```python
from build123d import *

# Parameters (mm, degrees)
F0_R        = 11.05
F1_DEPTH    = 6.5
F2_SIZE     = 2
F3_T1_DEPTH = 28.2168298797


# Not quite as in the source:
# - a fillet or chamfer that OpenCascade refuses, or shapes differently, is made with other operations: its cross-section is extruded or revolved along the edge and cut away or added


with BuildPart() as f1:
    # F0 (on Top) → F1 (new body)
    with BuildSketch(Plane.XY):
        Polygon((30, 0), (30, 15), (-30, 15), (-30, 0), (-30, -15), (30, -15), align=None)
        with BuildLine():
            ThreePointArc((-3.95, 0), (-15, -11.05), (-26.05, 0))
            ThreePointArc((-26.05, 0), (-15, 11.05), (-3.95, 0))
        make_face(mode=Mode.SUBTRACT)
        with Locations((15, 0)):
            Circle(F0_R, mode=Mode.SUBTRACT)
    extrude(amount=F1_DEPTH)

    # F2
    f2_edges = [f1.edges().sort_by_distance(p)[0] for p in [
        (-30, 0, 6.5),
        (-30, 0, 0),
        (0, -15, 0),
        (0, -15, 6.5),
        (0, 15, 0),
        (0, 15, 6.5),
        (30, 0, 0),
        (30, 0, 6.5),
    ]]
    chamfer(f2_edges, length=F2_SIZE)

    # F3: chamfer of 5 on 4 edges, made by hand

    # F3_s2 → F3_t1 (cut)
    with BuildSketch(Plane.XY.offset(-10.8584149398)):
        Polygon((30, 10), (25, 15), (30, 15), align=None)
        Polygon((30, -10), (25, -15), (30, -15), align=None)
        Polygon((-25, 15), (-30, 10), (-30, 15), align=None)
        Polygon((-25, -15), (-30, -10), (-30, -15), align=None)
    extrude(amount=F3_T1_DEPTH, mode=Mode.SUBTRACT)


solid = f1.part
```
For this review, take the finished solid that the model builds, in its own axes (mm). Give positions to 0.01 mm unless a question says otherwise; leave off trailing zeros. Write each loop counter-clockwise with the first axis right and the second up, starting at its lowest first coordinate (ties: lowest second). Pieces come first, ordered by that corner, then holes.
Item 1: Take a section at C-C (z = 5.75). Give the boundary of the cut face in (x, y).
Item 2: Take a section at D-D (y = -5). Give the boundary of the cut face in (x, z).
Item 3: Wall thickness on probe 1 along Y at (x, z) = (-15, 3); probe 2 along X at (y, z) = (-9.5, 5.5); probe 3 along X at (y, z) = (-8, 4.75): over which ranges is each line inside the solid? List them lowest first.
Item 4: Take a section at A-A (y = 0). Give the boundary of the cut face in (x, z), and give its area (3 significant figures).
Item 5: Take a section at B-B (x = -15). Give the boundary of the cut face in (y, z).
Item 6: Insertion check: P1, Ø1.5, axis at x = -5.5, z = 5.5, coming from the +Y side. The pin has a flat end and moves straight along its axis. Give the tip position at first contact, or say it passes through.
Established:
1. outline: (-28.75, -11.25) - (-26.25, -13.75) - (26.25, -13.75) - (28.75, -11.25) - (28.75, 11.25) - (26.25, 13.75) - (-26.25, 13.75) - (-28.75, 11.25) - close; hole circle Ø22.1 at (-15, 0); hole circle Ø22.1 at (15, 0)
2. outline: (-30, 2) - (-28, 0) - (-24.85, 0) - (-24.85, 6.5) - (-28, 6.5) - (-30, 4.5) - close; (-5.15, 0) - (5.15, 0) - (5.15, 6.5) - (-5.15, 6.5) - close; (24.85, 0) - (28, 0) - (30, 2) - (30, 4.5) - (28, 6.5) - (24.85, 6.5) - close
3. probe 1: y = -15 to -11.05, 11.05 to 15
3. probe 2: x = -29 to -20.64, -9.36 to 9.36, 20.64 to 29
3. probe 3: x = -29.75 to -22.62, -7.38 to 7.38, 22.62 to 29.75
4. outline: (-30, 2) - (-28, 0) - (-26.05, 0) - (-26.05, 6.5) - (-28, 6.5) - (-30, 4.5) - close; (-3.95, 0) - (3.95, 0) - (3.95, 6.5) - (-3.95, 6.5) - close; (26.05, 0) - (28, 0) - (30, 2) - (30, 4.5) - (28, 6.5) - (26.05, 6.5) - close
4. area: 94.7 mm2
5. outline: (-15, 2) - (-13, 0) - (-11.05, 0) - (-11.05, 6.5) - (-13, 6.5) - (-15, 4.5) - close; (11.05, 0) - (13, 0) - (15, 2) - (15, 4.5) - (13, 6.5) - (11.05, 6.5) - close
6. P1: stops at y = 14.75
